```python
from build123d import *

# Parameters (mm, degrees)
SKETCH1_R               = 11.25
BOSS_EXTRUDE1_DEPTH     = 33
FILLET1_R               = 5
CUT_EXTRUDE1_DEPTH      = 37.635024225
SKETCH3_OUTSIDE_W       = 29.846
SKETCH3_OUTSIDE_H       = 33.346
SKETCH3_OUTSIDE_R       = 7.9
CUT_EXTRUDE2_DEPTH      = 5
SKETCH4_R               = 5.8
CUT_EXTRUDE3_DEPTH      = 40.705950595
CUT_EXTRUDE4_REACH      = 38.136
CUT_EXTRUDE4_END_RADIUS = 5.8
SKETCH5_R               = 4.25


with BuildPart() as part:
    # Sketch1 → Boss-Extrude1 (new body)
    with BuildSketch(Plane(origin=(0, 0, 0), x_dir=(1, 0, 0), z_dir=(0, 1, 0))):
        with Locations(Location((0, 0, 0), (0, 0, 270))):
            Circle(SKETCH1_R)
    extrude(amount=BOSS_EXTRUDE1_DEPTH)

    # Fillet1
    fillet1_edges = [part.edges().sort_by_distance(p)[0] for p in [
        (0, 33, -11.25),
    ]]
    fillet(fillet1_edges, radius=FILLET1_R)

    # Sketch2 → Cut-Extrude1 (cut, through all)
    with BuildSketch(Plane(origin=(0, 33, 0), x_dir=(1, 0, 0), z_dir=(0, 1, 0))):
        with BuildLine():
            Line((-9.5, 6.025985397), (-9.5, -6.025985397))
            ThreePointArc((-9.5, -6.025985397), (-11.25, 0), (-9.5, 6.025985397))
        make_face()
        with BuildLine():
            Line((9.5, 6.025985397), (9.5, -6.025985397))
            ThreePointArc((9.5, -6.025985397), (11.25, 0), (9.5, 6.025985397))
        make_face()
    extrude(amount=-CUT_EXTRUDE1_DEPTH, mode=Mode.SUBTRACT)

    # Sketch3 outside → Cut-Extrude2 (cut)
    with BuildSketch(Plane.XZ):
        Rectangle(SKETCH3_OUTSIDE_W, SKETCH3_OUTSIDE_H)
        with Locations(Location((0, 0, 0), (0, 0, 270))):
            Circle(SKETCH3_OUTSIDE_R, mode=Mode.SUBTRACT)
    extrude(amount=-CUT_EXTRUDE2_DEPTH, mode=Mode.SUBTRACT)

    # Sketch4 → Cut-Extrude3 (cut, through all)
    with BuildSketch(Plane.ZY.offset(9.5)):
        with Locations((0, 21.7)):
            Circle(SKETCH4_R)
    extrude(amount=-CUT_EXTRUDE3_DEPTH, mode=Mode.SUBTRACT)

    # Cut-Extrude4: up to this cylinder (the profile starts outside it)
    cut_extrude4_end = Plane(origin=(0, 21.7, 0), z_dir=(-1, 0, 0)) * Cylinder(CUT_EXTRUDE4_END_RADIUS, 88.872, mode=Mode.PRIVATE)
    # Sketch5 → Cut-Extrude4 (cut, up to the surface)
    with BuildSketch(Plane.XZ, mode=Mode.PRIVATE) as cut_extrude4_sk1:
        with Locations(Location((0, 0, 0), (0, 0, 270))):
            Circle(SKETCH5_R)
    cut_extrude4_tool1 = extrude(cut_extrude4_sk1.sketch, amount=-CUT_EXTRUDE4_REACH, mode=Mode.PRIVATE) - cut_extrude4_end
    add(cut_extrude4_tool1.solids().sort_by_distance((0, 0, 0))[0], mode=Mode.SUBTRACT)


solid = part.part
```
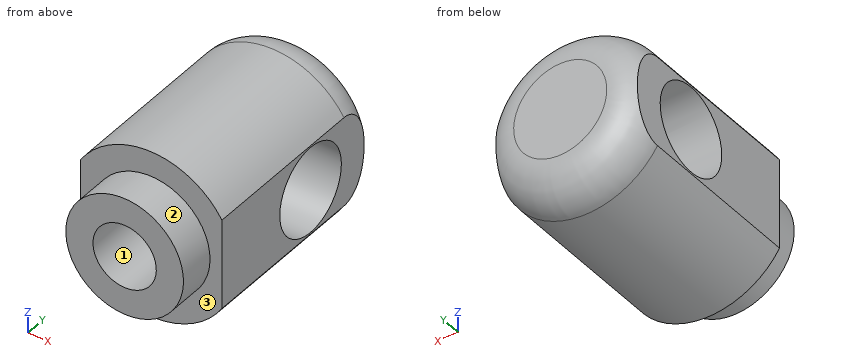
The listing builds one solid part. Answer for the finished solid, in the listing's coordinates (mm). Face numbers are marked on the shaded views. Give positions to 0.01 mm unless a question says otherwise; leave off trailing zeros. Order: outer loops, then holes, each group sorted by start corner. A loop starts at its lowest first (then second) coordinate and runs counter-clockwise, first axis right, second up. Notation, with made-up numbers: (63, -7) -> (120, -7) arc R17 cw to (120, 4) -> close; hole circle Ø7 at (27.5, -33.5). An arc over 180 degrees is marked (long way). Answer as a JSON object with one key per item and string values. Group by question number.
Item 1: The part is cut by section B-B on z = 0. Write down the section's boundary in (x, y).
Item 2: The part is cut by section D-D on y = 9.5. Write down the section's boundary in (x, z), and give its area (3 significant figures).
Item 3: The part is cut by section C-C on x = 0. Write down the section's boundary in (y, z), and give its area (3 significant figures).
Item 4: Consider L1, parallel to X at y = 8, z = 0; L2, parallel to Z at x = 0, y = 8.5; L3, parallel to Y at x = -5.5, z = 0. Determine where each line is inside the solid, lowest interval first. Write a range as from..to.
Item 5: The part is cut by section A-A on y = 21.7. Write down the section's boundary in (x, z).
Item 6: Determine the mould class of the marked faces 1, 2 and 3 for opening direction Z: pulls with the +Z half, pulls with the -Z half, needs draft (parallel to the pull), parting line crosses it, or undercut.
Item 7: Flat-ended cylindrical pins translate along their axes: pin 1 (2 mm diameter, centred on x = -2, y = 12.5, fed in from -Z); pin 2 (3 mm diameter, centred on x = -6, z = 6, fed in from +Y); pin 3 (5 mm diameter, centred on x = 7, y = 12, fed in from -Z). Find the tip coordinate at first contact, or state that the pin passes through.
Result set:
{
 "1": {"outline": "(-9.5, 5) -> (-7.9, 5) -> (-7.9, 0) -> (-4.25, 0) -> (-4.25, 15.9) -> (-9.5, 15.9) -> close; (-9.5, 27.5) -> (9.5, 27.5) -> (9.5, 31.8) arc R5 ccw to (6.25, 33) -> (-6.25, 33) arc R5 ccw to (-9.5, 31.8) -> close; (4.25, 0) -> (7.9, 0) -> (7.9, 5) -> (9.5, 5) -> (9.5, 15.9) -> (4.25, 15.9) -> close"},
 "2": {"outline": "(-9.5, -6.03) arc R11.25 ccw to (9.5, -6.03) -> (9.5, 6.03) arc R11.25 ccw to (-9.5, 6.03) -> close; hole circle Ø8.5 at (0, 0)", "area": "312 mm²"},
 "3": {"outline": "(0, -7.9) -> (5, -7.9) -> (5, -11.25) -> (28, -11.25) arc R5 ccw to (33, -6.25) -> (33, 6.25) arc R5 ccw to (28, 11.25) -> (5, 11.25) -> (5, 7.9) -> (0, 7.9) -> (0, 4.25) -> (17.75, 4.25) arc R5.8 cw (long way) to (17.75, -4.25) -> (0, -4.25) -> close", "area": "453 mm²"},
 "4": {"L1": "-9.5..-4.25, 4.25..9.5", "L2": "-11.25..-4.25, 4.25..11.25", "L3": "0..15.9, 27.5..33"},
 "5": {"outline": "(-9.5, -6.03) arc R11.25 ccw to (9.5, -6.03) -> (9.5, -5.8) -> (-9.5, -5.8) -> close; (-9.5, 5.8) -> (9.5, 5.8) -> (9.5, 6.03) arc R11.25 ccw to (-9.5, 6.03) -> close"},
 "6": {"face 1": "undercut", "face 2": "parting line crosses it", "face 3": "needs draft"},
 "7": {"pin 1": "z = -11.21", "pin 2": "y = 32.95", "pin 3": "z = -10.31"}
}
